Part model, mm, in its own coordinate system. A direction names the side the tool comes from. Give positions to 0.01 mm unless a question says otherwise; leave off trailing zeros. Order: outer loops, then holes, each group sorted by start corner. A loop starts at its lowest first (then second) coordinate and runs counter-clockwise, first axis right, second up.
from build123d import *

# Parameters (mm, degrees)
F1_DEPTH = 19.05
F2_W     = 19.05
F2_H     = 25.4
F3_DEPTH = 25.4
F4_W     = 19.05
F4_H     = 19.1262
F5_DEPTH = 6.35
F6_R     = 3.175
F7_DEPTH = 12.7


with BuildPart() as f1:
    # F0 (on Front) → F1 (new body)
    with BuildSketch(Plane.XZ):
        Polygon((0, 12.7), (0, 0), (6.35, 0), (6.35, 6.35), (19.05, 6.35), (19.05, 12.7), align=None)
    extrude(amount=-F1_DEPTH)

    # F2 (on Top) → F3 (join)
    with BuildSketch(Plane.XY):
        with Locations((28.575, 6.35)):
            Rectangle(F2_W, F2_H)
    extrude(amount=F3_DEPTH)

    # F4 (on face) → F5 (cut)
    with BuildSketch(Plane.XY.offset(25.4)):
        with Locations((28.575, 3.2131)):
            Rectangle(F4_W, F4_H)
    extrude(amount=-F5_DEPTH, mode=Mode.SUBTRACT)

    # F6 (on face) → F7 (cut, symmetric)
    with BuildSketch(Plane.XY.offset(12.7)):
        with Locations((28.575, 3.175)):
            Circle(F6_R)
        with Locations((9.525, 9.525)):
            Circle(F6_R)
    extrude(amount=F7_DEPTH, both=True, mode=Mode.SUBTRACT)


solid = f1.part
Item 1: Which spindle directions (+Z, -Z, +X, -X, +Y, -Y) get a long thin tool onto all of the face, cutting with end or side? Do faces 4 (the face through (24, 3, 19.05)), 5 (the face through (14, 9, 6.35)), 6 (the face through (7, 0, 8)), 7 (the face through (12, 7, 12.7)). Say none if no direction does.
Item 2: Drop flat-ended pins along their axis: P1, Ø6.5, axis at x = 10.5, z = 5, coming from the -Y side; P2, Ø6, axis at x = 21, y = -0.5, coming from the +Z side. Give the stop position or say it passes through.
Item 3: Band-saw the part on B-B on x = 27.5. List the corners of the cut face in (y, z), plus the area to 3 significant figures.
Item 4: Pull direction X, two halves, no side cores. Call faces 1 (the face through (28, 7, 0)), 2 (the face through (6.35, 9, 3)), 3 (the face through (0, 9, 6)): released by +X, released by -X, zero draft, split by the parting line, or undercut.
Item 5: Band-saw the part on C-C on y = 7.25. List the corners of the cut face in (x, z), plus the area to 3 significant figures.
Item 6: Band-saw the part on D-D on y = 14. List the corners of the cut face in (x, z).
Item 7: Band-saw the part on A-A on z = 4.75. List the corners of the cut face in (x, y) (3 decimals), plus the area to 3 significant figures.
Item 8: Drill centre lines: probe 1 along X at (y, z) = (9.5, 5.5); probe 2 along X at (y, z) = (0.25, 1.75); probe 3 along Z at (x, y) = (35, 11). Where is each one in solid material? Low to high.
Working result:
1. face 4: +Z, +X, -X, -Y
1. face 5: -Z, +Y, -Y
1. face 6: +Z, -Z, -X, -Y
1. face 7: +Z, -X, +Y, -Y
2. P1: stops at y = 0
2. P2: stops at z = 19.05
3. outline: (-6.35, 0) - (0.19, 0) - (0.19, 19.05) - (-6.35, 19.05) - close; (6.16, 0) - (19.05, 0) - (19.05, 25.4) - (12.78, 25.4) - (12.78, 19.05) - (6.16, 19.05) - close
3. area: 410 mm2
4. face 1: zero draft
4. face 2: undercut
4. face 3: released by -X
5. outline: (0, 0) - (6.35, 0) - (6.35, 6.35) - (7.31, 6.35) - (7.31, 12.7) - (0, 12.7) - close; (11.74, 6.35) - (19.05, 6.35) - (19.05, 0) - (38.1, 0) - (38.1, 19.05) - (19.05, 19.05) - (19.05, 12.7) - (11.74, 12.7) - close
5. area: 496 mm2
6. outline: (0, 0) - (6.35, 0) - (6.35, 6.35) - (19.05, 6.35) - (19.05, 0) - (38.1, 0) - (38.1, 25.4) - (19.05, 25.4) - (19.05, 12.7) - (0, 12.7) - close
7. outline: (0, 0) - (6.35, 0) - (6.35, 19.05) - (0, 19.05) - close; (19.05, -6.35) - (38.1, -6.35) - (38.1, 19.05) - (19.05, 19.05) - close; hole circle Ø6.35 at (28.575, 3.175)
7. area: 573 mm2
8. probe 1: x = 0 to 6.35, 19.05 to 38.1
8. probe 2: x = 0 to 6.35, 19.05 to 27.34, 29.81 to 38.1
8. probe 3: z = 0 to 19.05
